Autodesk Inventor part; units mm, degrees
ref_plane "Start plane" through (0, 0, 0) normal (0, 0, 1) x (1, 0, 0)
ref_plane "End plane" through (0, 0, 406.4) normal (0, 0, 1) x (1, 0, 0)
ref_plane "Work Plane4" through (0, 254, 406.4) normal (0, -1, 0) x (1, 0, 0)
ref_plane "Start plane" through (0, 0, 0) normal (0, 0, 1) x (1, 0, 0)
ref_plane "End plane" through (0, 0, 406.4) normal (0, 0, 1) x (1, 0, 0)
sketch "Sketch" plane through (0, 0, 0) normal (0, 0, 1) x (1, 0, 0)
  circle A0 centre (0, 0) radius 17.526
  circle A1 centre (0, 0) radius 21.082
  dimension "d0" = 42.164
  dimension "d1" = 3.556
extrude "Body" add sketch "Sketch" along normal up to surface (406.4 mm away) from surface at 0
sketch "Sketch3" plane through (0, 0, 0) normal (0, 0, 1) x (1, 0, 0)
  line L0 (0, 0) -> (10, 0)
ref_plane "Work Plane3" through (0, 0, 0) normal (0, -1, 0) x (1, 0, 0)
sketch "Sketch4" plane through (0, 0, 0) normal (0, -1, 0) x (1, 0, 0)
  line L0 (-2, 0) -> (12, 0)
  line L1 (-2, 406.4) -> (12, 406.4)
  dimension "d7" = 406.4
ref_plane "Work Plane4" through (0, 254, 406.4) normal (0, -1, 0) x (1, 0, 0)
ref_plane "Work Plane5" through (0, -1473.2, 406.4) normal (0, -1, 0) x (1, 0, 0)
ref_plane "Work Plane6" through (0, -609.6, 406.4) normal (0, -1, 0) x (1, 0, 0)
sketch "Sketch5" plane through (0, -609.6, 406.4) normal (0, -1, 0) x (1, 0, 0)
  circle A0 centre (0, 0) radius 21.082
  circle A1 centre (0, 0) radius 17.526
extrude "Extrusion2" cut sketch "Sketch5" along normal up to surface (1727.2 mm away) from surface at -863.6 contours A0 | A1
ref_plane "Work Plane7" through (0, -1473.2, 0) normal (0, 1, 0) x (1, 0, 0)
ref_plane "Work Plane8" through (0, 254, 0) normal (0, 1, 0) x (1, 0, 0)
ref_plane "Work Plane9" through (0, -609.6, 0) normal (0, 1, 0) x (1, 0, 0)
sketch "Sketch6" plane through (0, -609.6, 0) normal (0, 1, 0) x (1, 0, 0)
  circle A0 centre (0, 0) radius 21.082
  circle A1 centre (0, 0) radius 17.526
extrude "Extrusion3" cut sketch "Sketch6" along normal up to surface (1727.2 mm away) from surface at -863.6 contours A0 | A1
equation "\"d0\" = G_H"
equation "\"d1\" = G_T"
equation "\"d2\" = G_L"
equation "\"G_H\" = 42.164"
equation "\"G_T\" = 3.556"
equation "\"G_L\" = d7"
equation "\"G_OFFSET_START\" = 0"
equation "\"G_OFFSET_END\" = 0"
equation "\"d5\" = G_OFFSET_END + B_L"
equation "\"B_L\" = 406.4"
properties part number "ANSI - 1 1/4 x 0.140 - 16" material "Aluminum 6061"
Work out the finished part from the listing and answer in its coordinate system (mm). Coordinates: 2 decimals unless noted, no trailing zeros. Write each loop counter-clockwise with the first axis right and the second up, starting at its lowest first coordinate (ties: lowest second). Pieces come first, ordered by that corner, then holes. Notation, with made-up numbers: M 43,15 L 100,15 A25 ccw 100,39 Z; hole C 84,62 d9. An arc over 180 degrees is marked long. Use one line per item in the form item = value. Start each with the question number.
1. The mould has two halves that part along X. Classify faces 1 (the face through (-16.82, 6.17, 12.71)), 2 (the face through (20.11, -6.33, 200.36)), 3 (the face through (8.087, 15.549, 200.519)): released by +X, released by -X, zero draft, split by the parting line, or undercut.
2. The part is cut by section C-C (z = 219). Give the vertices of the cut face in (x, y).
3. The part is cut by section A-A (y = 0). Give the vertices of the cut face in (x, z).
4. The part is cut by section B-B (x = -10.5). Give the vertices of the cut face in (y, z), plus the area to 3 significant figures.
5. Each of these flat-tipped pins is pushed along its axis until it touches: P1, Ø12, axis at x = 8, z = 86, coming from the -Y side; P2, Ø2, axis at x = 4, z = 170, coming from the -Y side; P3, Ø8, axis at y = 7, z = 210, coming from the -X side; P4, Ø8, axis at x = 2, z = 256.5, coming from the -Y side. Where does it stop, or does it pass through?
6. Straight lines are drawn through the part: probe 1 along Y at (x, z) = (0, 88); probe 2 along Y at (x, z) = (10.5, 350). For each, find the intervals that lie inside material, in ascending order. Write a range as from..to.
Evaluation:
q1.face_1 = undercut
q1.face_2 = split by the parting line
q1.face_3 = undercut
q2.outline = C 0,0 d42.16; hole C 0,0 d35.05
q3.outline = M -21.08,0 A21.08 cw -17.53,11.72 L -17.53,394.68 A21.08 cw -21.08,406.4 Z; M 17.53,11.72 A21.08 cw 21.08,0 L 21.08,406.4 A21.08 cw 17.53,394.68 Z
q4.outline = M -18.28,18.28 L -14.03,18.28 L -14.03,388.12 L -18.28,388.12 Z; M 14.03,18.28 L 18.28,18.28 L 18.28,388.12 L 14.03,388.12 Z
q4.area = 3,140 mm^2
q5.P1 = -20.99
q5.P2 = -20.87
q5.P3 = -20.87
q5.P4 = -21.08
q6.probe_1 = -21.08..-17.53, 17.53..21.08
q6.probe_2 = -18.28..-14.03, 14.03..18.28
